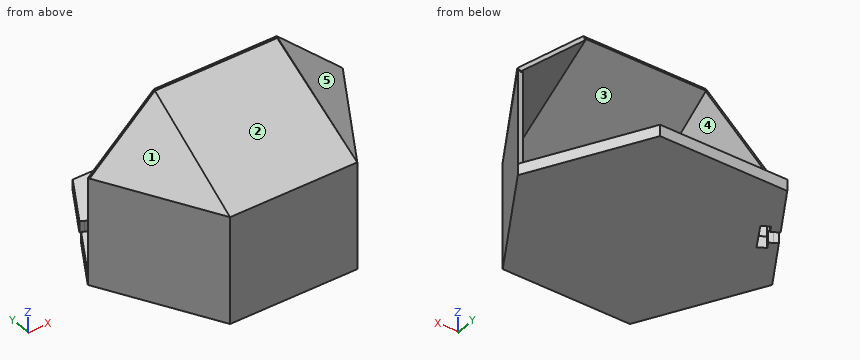
from build123d import *

# Parameters (mm, degrees)
F0_W      = 50
F0_H      = 12.5
F1_DEPTH  = 8
F2_DEPTH  = 75
F4_DEPTH  = 8
F7_DEPTH  = 3
F8_DEPTH  = 1
F11_DEPTH = 3
F14_DEPTH = 3
F15_DEPTH = 8
F16_DEPTH = 25
F17_DEPTH = 8


# Not quite as in the source:
# - a feature names something its author has since deleted; it is built from what else it names


with BuildPart() as f1:
    # F0 (on Top) → F1 (new body)
    with BuildSketch(Plane.XY):
        Polygon((-42.0179491924, 72.7772228311), (-60.5095952989, 40.7487522591), (-57.9695070384, 39.3207329262), (-55.5194165334, 43.6791064608), (-50.2642610162, 40.7248836223), (-52.7144317239, 36.366367418), (-57.615009792, 27.6494680496), (-60.0654171506, 23.2910848888), (-65.3204122546, 26.2455930623), (-62.870004896, 30.6039762231), (-65.5097997054, 32.0881441788), (-84.0358983849, 0), (-42.0179491924, -72.7772228311), (42.0179491924, -72.7772228311), (84.0358983849, 0), (42.0179491924, 72.7772228311), align=None)
        with Locations((0, 54.5829171234)):
            Rectangle(F0_W, F0_H, mode=Mode.SUBTRACT)
    extrude(amount=F1_DEPTH)

    # F0 (on Top) → F2 (join)
    with BuildSketch(Plane.XY):
        Polygon((43.75, -75.7772228311), (87.5, 0), (84.0358983849, 0), (42.0179491924, -72.7772228311), (-42.0179491924, -72.7772228311), (-84.0358983849, 0), (-87.5, 0), (-43.75, -75.7772228311), align=None)
    extrude(amount=F2_DEPTH)

    # F0 (on Top) → F4 (join)
    with BuildSketch(Plane.XY):
        Polygon((43.75, 75.7772228311), (-43.75, 75.7772228311), (-63.1248363216, 42.2190219338), (-60.5095952989, 40.7487522591), (-42.0179491924, 72.7772228311), (42.0179491924, 72.7772228311), (84.0358983849, 0), (87.5, 0), align=None)
    extrude(amount=F4_DEPTH)

    # F6 (on face) → F7 (join)
    with BuildSketch(Plane(origin=(0, -50.1312366318, 89.3836679776), x_dir=(1, 0, 0), z_dir=(0, 0.4891706574, -0.872188092))):
        Polygon((43.75, 29.4041920927), (0, 29.4041920927), (-43.75, 29.4041920927), (-42.01795, -57.4775522498), (42.01795, -57.4775522498), align=None)
    extrude(amount=F7_DEPTH)

    # F3 (on Front) → F8 (join)
    with BuildSketch(Plane.XZ):
        Polygon((-42.01795, 114.5), (0, 114.5), (42.01795, 114.5), (84.0359, 75), (87.5, 75), (42.01795, 117.5), (0, 117.5), (-42.01795, 117.5), (-87.5, 75), (-84.0359, 75), align=None)
    extrude(amount=F8_DEPTH)

    # F10 (on face) → F11 (join)
    with BuildSketch(Plane(origin=(-67.6846727043, -39.0777640058, 72.4338274863), x_dir=(0.7723629594, -0.3015876344, 0.5590173143), z_dir=(-0.6351814378, -0.3667221741, 0.6797495039))):
        Polygon((33.2314262259, 55.789645187), (-25.6554603702, 35.6104118215), (30.9888924807, -31.0804218073), align=None)
    extrude(amount=-F11_DEPTH)

    # F13 (on face) → F14 (join)
    with BuildSketch(Plane(origin=(67.6756688636, -39.5950852503, 72.4241918832), x_dir=(0.7733047167, 0.3041472681, -0.556322078), z_dir=(-0.6340345536, 0.3709553614, -0.6785221475))):
        Polygon((-30.939509805, 30.5117392321), (-32.8751652468, -56.3649154418), (25.9400068576, -35.9776056011), align=None)
    extrude(amount=F14_DEPTH)

    # F0 (on Top) → F15 (join)
    with BuildSketch(Plane.XY):
        with Locations((0, 54.5829171234)):
            Rectangle(F0_W, F0_H)
    extrude(amount=F15_DEPTH)

    # F0 (on Top) → F16 (cut)
    with BuildSketch(Plane.XY):
        Polygon((-57.9695070384, 39.3207329262), (-60.5095952989, 40.7487522591), (-65.5097997054, 32.0881441788), (-62.870004896, 30.6039762231), (-57.615009792, 27.6494680496), (-52.7144317239, 36.366367418), align=None)
    extrude(amount=-F16_DEPTH, mode=Mode.SUBTRACT)

    # F0 (on Top) → F17 (join)
    with BuildSketch(Plane.XY):
        Polygon((-65.5097997054, 32.0881441788), (-68.125, 33.5584843966), (-87.5, 0), (-84.0358983849, 0), align=None)
    extrude(amount=F17_DEPTH)


solid = f1.part
Model file for the job. Use its own axes, mm. Face numbers are marked on the shaded views. A direction names the side the tool comes from. Give positions to 0.01 mm unless a question says otherwise; leave off trailing zeros. Write each loop counter-clockwise with the first axis right and the second up, starting at its lowest first coordinate (ties: lowest second). Pieces come first, ordered by that corner, then holes. Notation, with made-up numbers: (-31.75, -14.5) -> (-10.75, -14.5) arc R18 ccw to (-10.75, -2.5) -> close; hole circle Ø9 at (46.5, -30.75). An arc over 180 degrees is marked (long way). Write item = value, one per line.
(1) Flat gauge pins, fed straight in: P1, Ø3, axis at y = -17, z = 31, coming from the -X side; P2, Ø1.5, axis at y = -3.5, z = 55, coming from the +X side; P3, Ø1.1, axis at x = -16, y = -0.5, coming from the +Z side. Where does each tip first touch, or does it go through?
Determined:
P1 = -78.55
P2 = 85.91
P3 = 117.5
(2) Slice it at D-D, the plane z = 94. Give the cut face in (x, y), then the cut area to 3 significant figures.
Determined:
outline = (-67.17, -1) -> (-66.59, -1) -> (-42.98, -41.9) -> (42.98, -41.9) -> (43.08, -42.16) -> (67.67, -0.14) -> (63.59, 0.98) -> (42.09, -35.77) -> (-41.79, -35.77) -> (-63.08, 1.1) -> (-67.17, 0) -> close
area = 894 mm2
(3) Slice it at B-B, the plane z = 18.5. Give the cut face in (x, y).
Determined:
outline = (-87.5, 0) -> (-43.75, -75.78) -> (43.75, -75.78) -> (87.5, 0) -> (84.04, 0) -> (42.02, -72.78) -> (-42.02, -72.78) -> (-84.04, 0) -> close
(4) Slice it at A-A, the plane x = -3. Give the cut face in (y, z), then the cut area to 3 significant figures.
Determined:
outline = (-75.78, 0) -> (75.78, 0) -> (75.78, 8) -> (-72.78, 8) -> (-72.78, 73.24) -> (1.47, 114.88) -> (0, 117.5) -> (-1, 117.5) -> (-1, 116.94) -> (-75.78, 75) -> close
area = 1,670 mm2
(5) Probe line 1 along Y through (x, z) = (-3, 43); line 2 along Z through (x, y) = (-61, 23.5); line 3 along X through (y, z) = (-50, 42.5). List the from-to ranges inside material, lowest first.
Determined:
line_1 = -75.78 to -72.78
line_2 = 0 to 8
line_3 = -58.63 to -55.17, 55.17 to 58.63
(6) Mould opens along X. For the marked faces 1, 2 and 3 say: released by +X, released by -X, zero draft, split by the parting line, or undercut.
Determined:
face_1 = released by -X
face_2 = zero draft
face_3 = undercut
(7) Tool access for the marked faces 4 and 5: list every direction of +Z, -Z, +X, -X, +Y, -Y with a clear straight run to the whole face (end or side of a thin tool).
Determined:
face_4 = +Y
face_5 = +Z, +X, -Y
(8) Slice it at C-C, the plane y = -28. Give the cut face in (x, z), then the cut area to 3 significant figures.
Determined:
outline = (-71.33, 0) -> (71.33, 0) -> (71.33, 75) -> (71.53, 75.16) -> (42.8, 102) -> (42.66, 101.8) -> (-42.66, 101.8) -> (-71.33, 75) -> close; hole (-67.87, 8) -> (67.87, 8) -> (67.87, 74.16) -> (41.98, 98.36) -> (-41.62, 98.36) -> (-67.87, 73.82) -> close
area = 2,130 mm2
